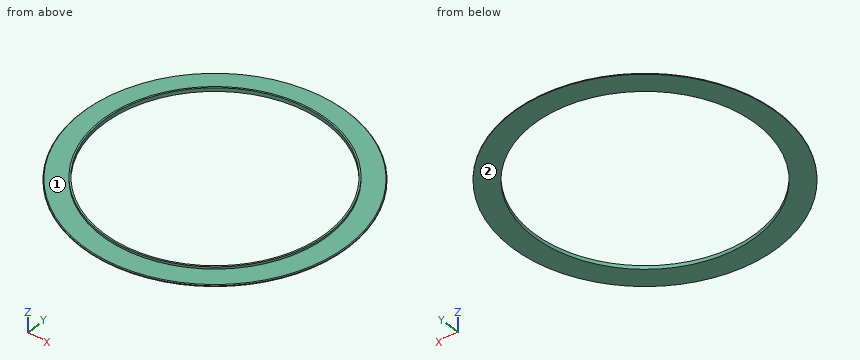
```python
from build123d import *

# Parameters (mm, degrees)
F0_R     = 37
F0_R_2   = 31.42
F0_R_3   = 31
F1_DEPTH = 0.4
F2_DEPTH = 1
F3_SIZE  = 0.2


with BuildPart() as f1:
    # F0 (on Top) → F1 (new body)
    with BuildSketch(Plane.XY):
        Circle(F0_R)
        Circle(F0_R_2, mode=Mode.SUBTRACT)
        Circle(F0_R_2)
        Circle(F0_R_3, mode=Mode.SUBTRACT)
    extrude(amount=F1_DEPTH)

    # F0 (on Top) → F2 (join)
    with BuildSketch(Plane.XY):
        Circle(F0_R_2)
        Circle(F0_R_3, mode=Mode.SUBTRACT)
    extrude(amount=F2_DEPTH)

    # F3
    f3_edges = [f1.edges().sort_by_distance(p)[0] for p in [
        (-37, 0, 0.4),
    ]]
    chamfer(f3_edges, length=F3_SIZE)


solid = f1.part
```
Input: part model. Units: mm. Frame: model coordinates. Face numbers are marked on the shaded views. A direction names the side the tool comes from. Round coordinates to 2 decimals unless told otherwise and drop trailing zeros. Order: outer loops, then holes, each group sorted by start corner. A loop starts at its lowest first (then second) coordinate and runs counter-clockwise, first axis right, second up. Notation, with made-up numbers: (61.5, -37.5) - (103.5, -37.5) arc R6 cw to (103.5, -29.5) - close; hole circle Ø6 at (71, -21). An arc over 180 degrees is marked (long way). One line per question, with ' | ' between items. Start each with the question number.
1) Ray query, probe 1 along Y at (x, z) = (0, 0.45); probe 2 along Z at (x, y) = (-14, -32); probe 3 along X at (y, z) = (-4.5, 0.9). Return the intervals inside material, ascending.
2) Set-up query: the marked faces 1 and 2. Return all of +Z, -Z, +X, -X, +Y, -Y with unobstructed straight access to the full face (end or side cutting, diameter ignored); none if empty.
3) Cut plane A-A, the plane y = 0. Return the cut outline in (x, z), then the cut area to 3 significant figures.
4) Contact query for flat-ended pins moving along their axis: P1, Ø22, axis at x = -16.5, y = 7.5, coming from the +Z side; P2, Ø12, axis at x = 23.5, y = -21.5, coming from the +Z side. Output: stop coordinate, or through.
5) Cut plane C-C, the plane z = 0.65. Return the cut outline in (x, y), then the cut area to 3 significant figures.
Worked out:
1) probe 1: y = -31.42 to -31, 31 to 31.42 | probe 2: z = 0 to 0.4 | probe 3: x = -31.1 to -30.67, 30.67 to 31.1
2) face 1: +Z | face 2: -Z, +X, -X, +Y, -Y
3) outline: (-37, 0) - (-31, 0) - (-31, 1) - (-31.42, 1) - (-31.42, 0.4) - (-36.8, 0.4) - (-37, 0.2) - close; (31, 0) - (37, 0) - (37, 0.2) - (36.8, 0.4) - (31.42, 0.4) - (31.42, 1) - (31, 1) - close | area: 5.26 mm^2
4) P1: passes through | P2: stops at z = 1
5) outline: circle Ø62.84 at (0, 0); hole circle Ø62 at (0, 0) | area: 82.4 mm^2
